```python
from build123d import *

# Parameters (mm, degrees)
SKETCH_W      = 48
SKETCH_H      = 54
PAD_DEPTH     = 2
SKETCH001_R   = 1.4
PAD001_DEPTH  = 2
SKETCH002_R   = 3.4
SKETCH002_R_2 = 1.4
PAD002_DEPTH  = 2
SKETCH003_R   = 1.4
PAD003_DEPTH  = 5
SKETCH004_R   = 1.4
PAD004_DEPTH  = 5


with BuildPart() as body:
    # Sketch → Pad (new body)
    with BuildSketch(Plane.XZ):
        Rectangle(SKETCH_W, SKETCH_H)
    extrude(amount=PAD_DEPTH)

    # Sketch001 (on Face2 of Pad) → Pad001 (join)
    with BuildSketch(Plane(origin=(24, 0, 0), x_dir=(0, 0, 1), z_dir=(1, 0, 0))):
        with BuildLine():
            Line((-27.5, 0), (27.5, 0))
            ThreePointArc((27.5, 0), (32.5, 5), (27.5, 10))
            ThreePointArc((22.5, 15), (23.964466, 11.464466), (27.5, 10))
            Line((22.5, 35.980762), (22.5, 15))
            ThreePointArc((22.5, 35.980762), (21.035534, 39.516296), (17.5, 40.980762))
            Line((17.5, 40.980762), (-17.5, 40.980762))
            ThreePointArc((-17.5, 40.980762), (-21.035534, 39.516296), (-22.5, 35.980762))
            Line((-22.5, 35.980762), (-22.5, 15))
            ThreePointArc((-27.5, 10), (-23.964466, 11.464466), (-22.5, 15))
            ThreePointArc((-27.5, 10), (-32.5, 5), (-27.5, 0))
        make_face()
        with Locations((-27.5, 5)):
            Circle(SKETCH001_R, mode=Mode.SUBTRACT)
        with Locations((27.5, 5)):
            Circle(SKETCH001_R, mode=Mode.SUBTRACT)
        with Locations((12.5, 30.980762)):
            Circle(SKETCH001_R, mode=Mode.SUBTRACT)
        with Locations((17.5, 25.980762)):
            Circle(SKETCH001_R, mode=Mode.SUBTRACT)
        with Locations((17.5, 35.980762)):
            Circle(SKETCH001_R, mode=Mode.SUBTRACT)
        with Locations((7.5, 35.980762)):
            Circle(SKETCH001_R, mode=Mode.SUBTRACT)
        with Locations((7.5, 25.980762)):
            Circle(SKETCH001_R, mode=Mode.SUBTRACT)
        with Locations((-12.5, 30.980762)):
            Circle(SKETCH001_R, mode=Mode.SUBTRACT)
    extrude(amount=PAD001_DEPTH)

    # Sketch002 (on Face4 of Pad) → Pad002 (join)
    with BuildSketch(Plane(origin=(-24, 0, 0), x_dir=(0, 0, -1), z_dir=(-1, 0, 0))):
        with BuildLine():
            Line((27, 0), (-27, 0))
            ThreePointArc((-27.5, 10.024938), (-32.518699, 4.749689), (-27, 0))
            ThreePointArc((-27.5, 10.024938), (-23.964466, 11.489404), (-22.5, 15.024938))
            Line((-22.5, 35.980762), (-22.5, 15.024938))
            ThreePointArc((-17.5, 40.980762), (-21.035534, 39.516296), (-22.5, 35.980762))
            Line((-17.5, 40.980762), (17.5, 40.980762))
            ThreePointArc((22.5, 35.980762), (21.035534, 39.516296), (17.5, 40.980762))
            Line((22.5, 35.980762), (22.5, 15.024938))
            ThreePointArc((22.5, 15.024938), (23.964466, 11.489404), (27.5, 10.024938))
            ThreePointArc((27, 0), (32.518699, 4.749689), (27.5, 10.024938))
        make_face()
        with Locations((-12.5, 30.980762)):
            Circle(SKETCH002_R, mode=Mode.SUBTRACT)
        with Locations((12.5, 30.980762)):
            Circle(SKETCH002_R_2, mode=Mode.SUBTRACT)
        with Locations((27.5, 5)):
            Circle(SKETCH002_R_2, mode=Mode.SUBTRACT)
        with Locations((-27.5, 5)):
            Circle(SKETCH002_R_2, mode=Mode.SUBTRACT)
    extrude(amount=PAD002_DEPTH)

    # Sketch003 (on Face26 of Pad002) → Pad003 (join)
    with BuildSketch(Plane(origin=(-24, 0, 0), x_dir=(0, 0, 1), z_dir=(1, 0, 0))):
        with BuildLine():
            ThreePointArc((-27.5, 10), (-32.5, 5), (-27.5, 0))
            Line((27, 0), (-27.5, 0))
            ThreePointArc((27, 0), (32.518699, 4.749689), (27.5, 10.024938))
            Line((-27.5, 10), (27.5, 10.024938))
        make_face()
        with Locations((-27.5, 5)):
            Circle(SKETCH003_R, mode=Mode.SUBTRACT)
        with Locations((27.5, 5)):
            Circle(SKETCH003_R, mode=Mode.SUBTRACT)
    extrude(amount=PAD003_DEPTH)

    # Sketch004 (on Face4 of Pad003) → Pad004 (join)
    with BuildSketch(Plane(origin=(24, 0, 0), x_dir=(0, 0, -1), z_dir=(-1, 0, 0))):
        with BuildLine():
            ThreePointArc((-27.5, 10), (-32.5, 5), (-27.5, 0))
            Line((27.5, 0), (-27.5, 0))
            ThreePointArc((27.5, 0), (32.5, 5), (27.5, 10))
            Line((22.5, 10), (27.5, 10))
            ThreePointArc((17.5, 15), (18.964466, 11.464466), (22.5, 10))
            Line((17.5, 30.980762), (17.5, 15))
            ThreePointArc((17.5, 30.980762), (12.5, 35.980762), (7.5, 30.980762))
            Line((7.5, 30.980762), (7.5, 15))
            ThreePointArc((2.5, 10), (6.035534, 11.464466), (7.5, 15))
            Line((-27.5, 10), (2.5, 10))
        make_face()
        with Locations((-27.5, 5)):
            Circle(SKETCH004_R, mode=Mode.SUBTRACT)
        with Locations((27.5, 5)):
            Circle(SKETCH004_R, mode=Mode.SUBTRACT)
        with Locations((12.5, 30.980762)):
            Circle(SKETCH004_R, mode=Mode.SUBTRACT)
    extrude(amount=PAD004_DEPTH)


with BuildPart() as part_mirroring:
    # Part__Mirroring: instance of Body
    add(body.part.mirror(Plane(origin=(0, 0, 0), x_dir=(0, -1, 0), z_dir=(1, 0, 0))))


solid = part_mirroring.part
```
Here's how the part is built. I have some questions about the finished solid (model axes, mm). A direction names the side the tool comes from. Give positions to 0.01 mm unless a question says otherwise; leave off trailing zeros. Loops run counter-clockwise (first coordinate to the right, second up) from the corner with the lowest first, then second, coordinate; pieces in that order, holes last. Notation, with made-up numbers: M -16,-1.5 L -10,-1.5 A13 cw -10,12.5 Z; hole C -9.5,15 d5. An arc over 180 degrees is marked long. Put each result on its own line as item: value. Start each with the question number.
(1) I want a section at A-A on y = -22.5. Please give me the cut outline in (x, z).
(2) I need wall thicknesses on line 1 along Z through (x, y) = (-25, -5); line 2 along X through (y, z) = (-3.5, -2.5); line 3 along Y through (x, z) = (22.75, 27.5). Which ranges of each line are inside material? Lowest first, please. Write a range as [from, to].
(3) If we mould it in two halves opening along X, with no side actions, what happens to faces 4 (the cylindrical face through (-21.54, -11.5, -18.93)), 5 (the cylindrical face through (-21.54, -35.98, -12.61)), 6 (the cylindrical face through (-25, -26, 16.1))? For each: +X half, -X half, draft (parallel to the pull), parting line (faces both ways), or undercut.
(4) I want a section at B-B on x = -21.5. Please give me the cut outline in (y, z), then the cut area to 3 significant figures.
(5) I want a section at D-D on y = -11.5. Please give me the cut outline in (x, z).
(6) Will these pins go through, and if not, where does the flat tip stop? pin 1 Ø4.5 at (y, z) = (-30.98, 12.5) entering from +X; pin 2 Ø3 at (x, z) = (7.5, -18) entering from -Y; pin 3 Ø2 at (x, z) = (4.5, 13) entering from +Y.
(7) I want a section at C-C on z = 7.5. Please give me the cut outline in (x, y), then the cut area to 3 significant figures.
(8) For faces 1 (the cylindrical face through (-24.986, -34.614, 7.197)), 2 (the flat face through (-22, -23, -7.5)), 3 (the flat face through (-25, -26, -22.5)), which set-ups out of +Z, -Z, +X, -X, +Y, -Y let a thin tool reach every point of the face, with its end or its side?
Answer block:
1. outline: M -26,-22.5 L -24,-22.5 L -24,-17.5 L -19,-17.5 L -19,-7.5 L -24,-7.5 L -24,22.5 L -26,22.5 Z; M 24,-22.5 L 26,-22.5 L 26,22.5 L 24,22.5 Z
2. line 1: [-32.5, -28.9], [-26.1, 26.1], [28.9, 32.5]
2. line 2: [-26, -19], [19, 26]
2. line 3: [-10.02, -6.4], [-3.6, 0.02]
3. face 4: undercut
3. face 5: undercut
3. face 6: draft
4. outline: M -30.98,-17.5 L -15,-17.5 A5 cw -10,-22.5 L -10,-27.5 A5 ccw 0,-27.5 L 0,27.5 A5 ccw -10,27.5 L -10,-2.5 A5 cw -15,-7.5 L -30.98,-7.5 A5 ccw Z; hole C -30.98,-12.5 d2.8; hole C -5,-27.5 d2.8; hole C -5,27.5 d2.8
4. area: 870 mm^2
5. outline: M -26,-23.93 L -24,-23.93 L -24,-18.93 L -19,-18.93 L -19,-6.07 L -24,-6.07 L -24,23.93 L -26,23.93 Z; M 24,-23.95 L 26,-23.95 L 26,23.95 L 24,23.95 Z
6. pin 1: x = -24
6. pin 2: y = -2
6. pin 3: y = 0
7. outline: M -26,-40.98 L -24,-40.98 L -24,-37.38 L -26,-37.38 Z; M -26,-34.58 L -24,-34.58 L -24,-27.38 L -26,-27.38 Z; M -26,-24.58 L -24,-24.58 L -24,-10 L -19,-10 L -19,-2 L 19,-2 L 19,-10.02 L 24,-10.02 L 24,-40.98 L 26,-40.98 L 26,0 L -26,0 Z
7. area: 329 mm^2
8. face 1: -X
8. face 2: +Z, -Y
8. face 3: -Z, +X, -X, -Y
